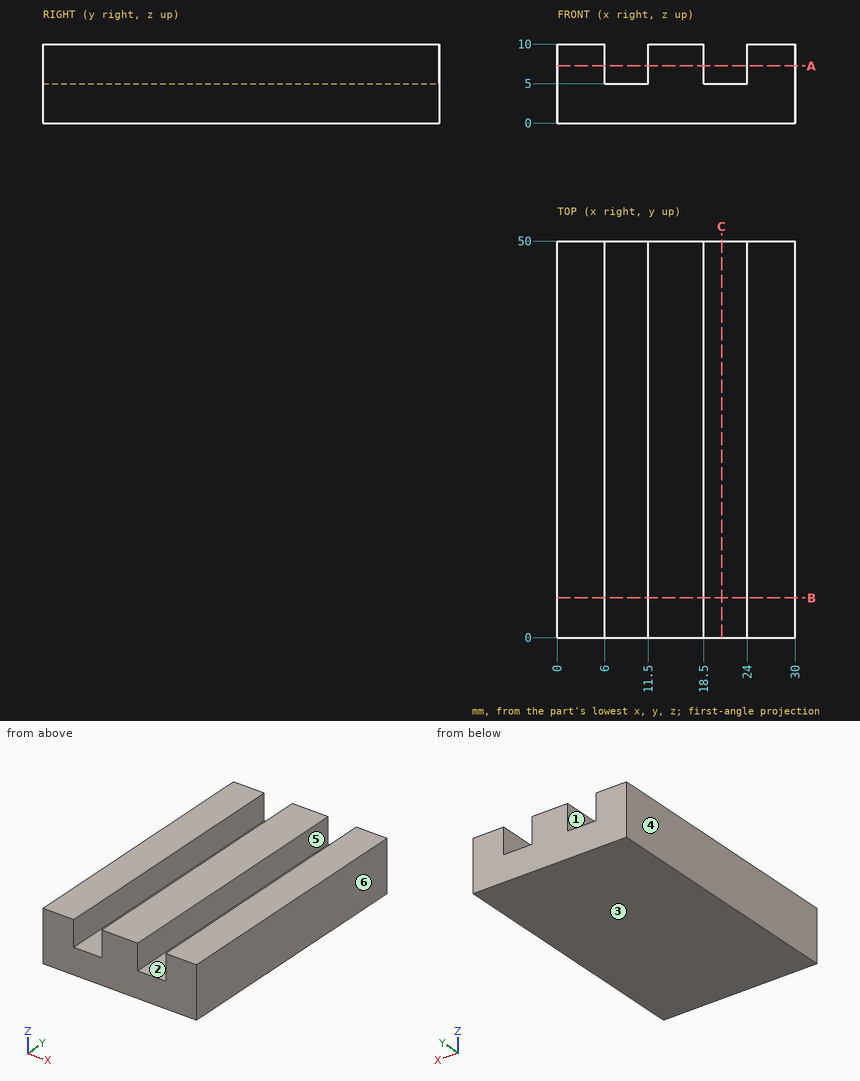
Could you check a few things on this drawing? It's one solid part, dimensions in mm from its lowest x, y, z. A direction names the side the tool comes from. Give positions to 0.01 mm unless a question says otherwise; leave off trailing zeros. Loops run counter-clockwise (first coordinate to the right, second up) from the corner with the lowest first, then second, coordinate; pieces in that order, holes last. Notation, with made-up numbers: (-39, -28) -> (-9, -28) arc R7 cw to (-9, -16) -> close; hole circle Ø6 at (70, 80.5). An arc over 180 degrees is marked (long way). Answer as CSV lines item,"result". Start each with the question number.
(1) If we section it at C-C on x = 20.75: Write out the boundary of the cut face in (y, z), then the cut area to 3 significant figures.
(2) If we section it at B-B on y = 5: Write out the boundary of the cut face in (x, z).
(3) If we section it at A-A on z = 7.25: Write out the boundary of the cut face in (x, y).
(4) Which directions (+Z, -Z, +X, -X, +Y, -Y) give clear straight access to the entire face, cutting with the end or side of a thin tool? Please do the marked faces 5 and 6.
(5) We'd pull the mould along X, two halves only. Please class the marked faces 1, 2, 3 and 4: released by +X, released by -X, zero draft, split by the parting line, or undercut.
(6) I'm going to push flat-ended pins straight in: pin 1 Ø5.5 at (y, z) = (32.5, 8) entering from -X; pin 2 Ø3 at (x, z) = (21, 9) entering from -Y; pin 3 Ø1.6 at (x, y) = (9, 22) entering from +Z. Where does each tip first touch, or does it pass through?
(7) I need wall thicknesses on probe 1 along X at (y, z) = (44, 8.5); probe 2 along Z at (x, y) = (21.25, 9.5). Which ranges of each line are inside material? Lowest first, please.
Computed:
1,outline,"(0, 0) -> (50, 0) -> (50, 5) -> (0, 5) -> close"
1,area,"250 mm2"
2,outline,"(0, 0) -> (30, 0) -> (30, 10) -> (24, 10) -> (24, 5) -> (18.5, 5) -> (18.5, 10) -> (11.5, 10) -> (11.5, 5) -> (6, 5) -> (6, 10) -> (0, 10) -> close"
3,outline,"(0, 0) -> (6, 0) -> (6, 50) -> (0, 50) -> close; (11.5, 0) -> (18.5, 0) -> (18.5, 50) -> (11.5, 50) -> close; (24, 0) -> (30, 0) -> (30, 50) -> (24, 50) -> close"
4,face 5,"+Z, +Y, -Y"
4,face 6,"+Z, -Z, +X, +Y, -Y"
5,face 1,"undercut"
5,face 2,"undercut"
5,face 3,"zero draft"
5,face 4,"released by -X"
6,pin 1,"stops at x = 0"
6,pin 2,"passes through"
6,pin 3,"stops at z = 5"
7,probe 1,"x = 0 to 6, 11.5 to 18.5, 24 to 30"
7,probe 2,"z = 0 to 5"
